Job drawing, mm, ordinate dimensions from the low corner. One solid piece. Give positions to 0.01 mm unless a question says otherwise; leave off trailing zeros. Write each loop counter-clockwise with the first axis right and the second up, starting at its lowest first coordinate (ties: lowest second). Pieces come first, ordered by that corner, then holes. Notation, with made-up numbers: M -28,23 L 6,23 A32 cw 6,52 Z; hole C 43.25,-16 d8. An arc over 180 degrees is marked long. Use CSV: the item, a comma, the result in double quotes. Start each with the question number.
Item 1: Cut at D-D (y = 1.5). List the corners of the cut face in (x, z) (1 decimal).
Item 2: Cut at C-C (z = 4). List the corners of the cut face in (x, y) (1 decimal).
Item 3: Cut at B-B (x = 6.25). List the corners of the cut face in (y, z).
Item 4: Mould opens along Y. For the marked faces 1, 2 and 3 say: released by +Y, released by -Y, zero draft, split by the parting line, or undercut.
Item 5: Pin check, flat tips, straight feed: pin 1 (3 mm diameter, centred on y = 2, z = 10.5, fed in from +X); pin 2 (2 mm diameter, centred on y = 5.5, z = 17.5, fed in from -X); pin 3 (2.5 mm diameter, centred on x = 3.97, y = 3.97, fed in from -Z). Stop position of each tip, or through.
Item 6: Cut at A-A (x = 4). List the corners of the cut face in (y, z) (1 decimal).
Item 7: Drill centre lines: line 1 (Y direction, x = 4, z = 8.25) (1 decimal); line 2 (Z direction, x = 4, y = 6); line 3 (Z direction, x = 5.25, y = 0.5). Where is each one in solid material? Low to high. Write a range as [from, to].
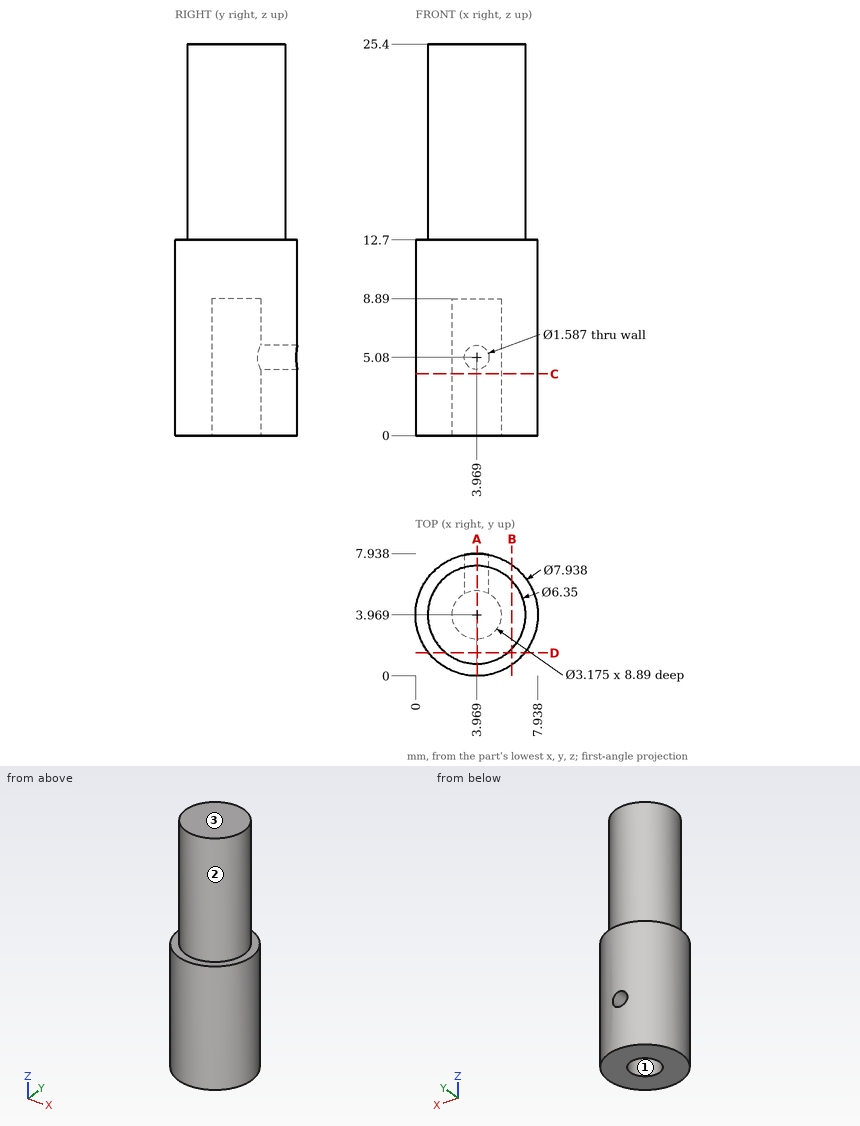
Worked answers:
1,outline,"M 0.9,0 L 7.1,0 L 7.1,12.7 L 6,12.7 L 6,25.4 L 2,25.4 L 2,12.7 L 0.9,12.7 Z"
2,outline,"C 4,4 d7.9; hole C 4,4 d3.2"
3,outline,"M 0.72,0 L 7.22,0 L 7.22,12.7 L 6.18,12.7 L 6.18,25.4 L 1.76,25.4 L 1.76,12.7 L 0.72,12.7 Z"
4,face 1,"undercut"
4,face 2,"split by the parting line"
4,face 3,"zero draft"
5,pin 1,"stops at x = 7.91"
5,pin 2,"stops at x = 0.84"
5,pin 3,"stops at z = 8.89"
6,outline,"M 0,0 L 2.4,0 L 2.4,8.9 L 5.6,8.9 L 5.6,5.9 L 7.9,5.9 L 7.9,12.7 L 7.1,12.7 L 7.1,25.4 L 0.8,25.4 L 0.8,12.7 L 0,12.7 Z; M 5.6,0 L 7.9,0 L 7.9,4.3 L 5.6,4.3 Z"
7,line 1,"y = [0, 2.4], [5.6, 7.9]"
7,line 2,"z = [0, 4.29], [5.87, 25.4]"
7,line 3,"z = [0, 12.7]"
